from build123d import *

# Parameters (mm, degrees)
SKETCH1_R                                     = 76.2
BOSS_EXTRUDE1_DEPTH                           = 25.4
CBORE_FOR_1_4_BUTTON_HEAD_CAP_SCREW2_AT_COUNT = 2
CBORE_FOR_1_4_BUTTON_HEAD_CAP_SCREW2_AT_PITCH = 48.170302877
CBORE_FOR_1_4_BUTTON_HEAD_CAP_SCREW2_2_COUNT  = 2
CBORE_FOR_1_4_BUTTON_HEAD_CAP_SCREW2_2_PITCH  = 68.123095633
CBORE_FOR_1_4_BUTTON_HEAD_CAP_SCREW2_3_COUNT  = 2
CBORE_FOR_1_4_BUTTON_HEAD_CAP_SCREW2_3_PITCH  = 48.170302877
CIRPATTERN1_COUNT                             = 12


with BuildPart() as part:
    # Sketch1 → Boss-Extrude1 (new body)
    with BuildSketch(Plane(origin=(0, 0, 0), x_dir=(1, 0, 0), z_dir=(0, 1, 0))):
        with Locations(Location((0, 0, 0), (0, 0, 270))):
            Circle(SKETCH1_R)
    extrude(amount=-BOSS_EXTRUDE1_DEPTH)

    # Sketch13 → CBORE for 1/4 Button Head Cap Screw2 (revolve, cut)
    with BuildSketch(Plane(origin=(-34.061547816, 0, 0), x_dir=(0, 0, 1), z_dir=(1, 0, 0))):
        Polygon((0, 0), (0, 25.4), (3.3782, 25.4), (3.3782, 3.3528), (5.95376, 3.3528), (5.95376, 0.635), (6.58876, 0), align=None)
    cbore_for_1_4_button_head_cap_screw2 = revolve(axis=Axis((-34.061547816, 6.35, 0), (0, -1, 0)), mode=Mode.SUBTRACT)

    # CBORE for 1/4 Button Head Cap Screw2 at: CBORE for 1/4 Button Head Cap Screw2 ×2
    with Locations(*[Vector(0.7071067811865476, 0, -0.7071067811865476) * (i * CBORE_FOR_1_4_BUTTON_HEAD_CAP_SCREW2_AT_PITCH) for i in range(1, CBORE_FOR_1_4_BUTTON_HEAD_CAP_SCREW2_AT_COUNT)]):
        add(cbore_for_1_4_button_head_cap_screw2, mode=Mode.SUBTRACT)

    # CBORE for 1_4 Button Head Cap Screw2 2: CBORE for 1/4 Button Head Cap Screw2 ×2
    with Locations(*[(i * CBORE_FOR_1_4_BUTTON_HEAD_CAP_SCREW2_2_PITCH, 0, 0) for i in range(1, CBORE_FOR_1_4_BUTTON_HEAD_CAP_SCREW2_2_COUNT)]):
        add(cbore_for_1_4_button_head_cap_screw2, mode=Mode.SUBTRACT)

    # CBORE for 1_4 Button Head Cap Screw2 3: CBORE for 1/4 Button Head Cap Screw2 ×2
    with Locations(*[Vector(0.7071067811865476, 0, 0.7071067811865476) * (i * CBORE_FOR_1_4_BUTTON_HEAD_CAP_SCREW2_3_PITCH) for i in range(1, CBORE_FOR_1_4_BUTTON_HEAD_CAP_SCREW2_3_COUNT)]):
        add(cbore_for_1_4_button_head_cap_screw2, mode=Mode.SUBTRACT)

    # Sketch16 → CBORE for 1/4 Button Head Cap Screw3 (revolve, cut)
    with BuildSketch(Plane(origin=(63.5, 0, 0), x_dir=(0, 0, 1), z_dir=(1, 0, 0))):
        Polygon((0, 0), (0, 25.4), (3.3782, 25.4), (3.3782, 3.3528), (5.95376, 3.3528), (5.95376, 0.635), (6.58876, 0), align=None)
    cbore_for_1_4_button_head_cap_screw3 = revolve(axis=Axis((63.5, 6.35, 0), (0, -1, 0)), mode=Mode.SUBTRACT)

    # CirPattern1: CBORE for 1/4 Button Head Cap Screw3 ×12 about axis
    cirpattern1_axis = Axis((0, 0, 0), (0, 1, 0))
    for i in range(1, CIRPATTERN1_COUNT):
        add(cbore_for_1_4_button_head_cap_screw3.rotate(cirpattern1_axis, i * 360 / CIRPATTERN1_COUNT), mode=Mode.SUBTRACT)


solid = part.part
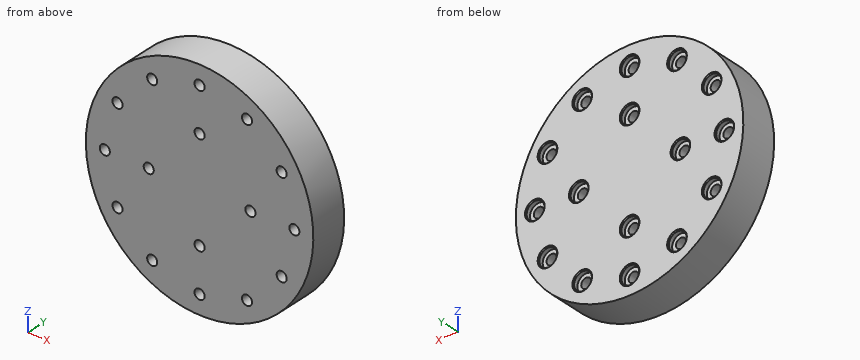
Build history of the part. All positions in model axes, mm. Round coordinates to 2 decimals unless told otherwise and drop trailing zeros. Loops run counter-clockwise (first coordinate to the right, second up) from the corner with the lowest first, then second, coordinate; pieces in that order, holes last. Notation, with made-up numbers: (63, 56) -> (120, 56) arc R38 cw to (120, 94) -> close; hole circle Ø8 at (12, 4.25). An arc over 180 degrees is marked (long way). Answer in a Markdown table with one row per item.
Item 1: Saw through at A-A (x = 63.5). Write the cut outline in (y, z) (3 decimals).
Answers below:
| item | result |
|---|---|
| outline | (-25.4, -42.121) -> (0, -42.121) -> (0, -6.589) -> (-0.635, -5.954) -> (-3.353, -5.954) -> (-3.353, -3.378) -> (-25.4, -3.378) -> close; (-25.4, 3.378) -> (-3.353, 3.378) -> (-3.353, 5.954) -> (-0.635, 5.954) -> (0, 6.589) -> (0, 42.121) -> (-25.4, 42.121) -> close |
Item 2: Saw through at C-C (y = -21.25). State how many separate pieces and enclosed holes the cut face has, and give its area (3 significant figures).
Answers below:
| item | result |
|---|---|
| separate pieces | 1 |
| enclosed holes | 16 |
| area | 17,700 mm² |
Item 3: Drill centre lines: L1, parallel to X at y = -8.5, z = 0; L2, parallel to X at y = -10.75, z = 57.5; L3, parallel to Y at x = -54, z = -36. Where is each one in solid material? Low to high. Write a range as [from, to].
Answers below:
| item | result |
|---|---|
| L1 | x = [-76.2, -66.88], [-60.12, -37.44], [-30.68, 30.68], [37.44, 60.12], [66.88, 76.2] |
| L2 | x = [-50, -34.01], [-29.49, 29.49], [34.01, 50] |
| L3 | y = [-25.4, -3.35] |
Item 4: Pin check, flat tips, straight feed: pin 1 (11 mm diameter, centred on x = 0, z = 34.06, fed in from +Y); pin 2 (2 mm diameter, centred on x = 3, y = -10, fed in from -Z); pin 3 (3.5 mm diameter, centred on x = 0.5, z = 65, fed in from +Y); pin 4 (2 mm diameter, centred on y = -9, z = 48.5, fed in from +X). Stop position of each tip, or through.
Answers below:
| item | result |
|---|---|
| pin 1 | stops at y = -3.35 |
| pin 2 | stops at z = -76.17 |
| pin 3 | passes through |
| pin 4 | stops at x = 59.58 |
Item 5: Saw through at B-B (z = 63.5). Write the cut outline in (x, y) (3 decimals), and give its area (3 significant figures).
Answers below:
| item | result |
|---|---|
| outline | (-42.121, -25.4) -> (-3.378, -25.4) -> (-3.378, -3.353) -> (-5.954, -3.353) -> (-5.954, -0.635) -> (-6.589, 0) -> (-42.121, 0) -> close; (3.378, -25.4) -> (42.121, -25.4) -> (42.121, 0) -> (6.589, 0) -> (5.954, -0.635) -> (5.954, -3.353) -> (3.378, -3.353) -> close |
| area | 1,950 mm² |
